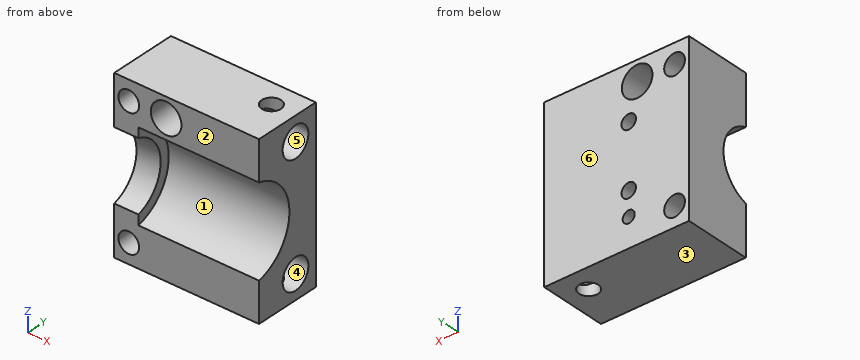
Autodesk Inventor part; units mm, degrees
ref_plane "YZ Plane" through (0, 0, 0) normal (1, 0, 0) x (0, 1, 0)
ref_plane "XZ Plane" through (0, 0, 0) normal (0, 1, 0) x (-1, 0, 0)
ref_plane "XY Plane" through (0, 0, 0) normal (0, 0, 1) x (1, 0, 0)
sketch "Sketch1" plane through (0, 0, 0) normal (0, 0, 1) x (1, 0, 0)
  line L0 (15, -7) -> (-15, -7)
  line L1 (-15, -7) -> (-15, 7)
  line L2 (-15, 7) -> (15, 7)
  line L3 (15, 7) -> (15, -7)
  line L4 (15, -7) -> (-15, 7) construction
  line L5 (-15, -7) -> (15, 7) construction
  point P0 (0, 0)
  dimension "d0" = 30
  dimension "d1" = 14
extrude "Extrusion1" add sketch "Sketch1" along normal blind 35
sketch "Sketch3" plane through (15, -7, 0) normal (1, 0, 0) x (0, 0, -1)
  line L0 (0, 0) -> (-35, 0)
  line L1 (-17.5, 0) -> (-17.5, -2)
  arc A0 (-8.2129, 0) -> (-26.7871, 0) centre (-17.5, -2) ccw
  point P0 (0, 7)
  dimension "d4" = 2
  dimension "d5" = 19
extrude "Extrusion2" cut sketch "Sketch3" against normal blind 25
sketch "Sketch5" plane through (-15, 7, 0) normal (0, 1, 0) x (1, 0, 0)
  line L0 (30, 0) -> (0, 0)
  line L1 (30, -35) -> (0, -35)
  line L2 (0, -35) -> (0, -30.9)
  line L3 (0, 0) -> (0, -35)
  line L4 (0, -30.9) -> (2.75, -30.9)
  circle A0 centre (2.75, -30.9) radius 2
  line L5 (0, 0) -> (0, -4.1)
  line L6 (0, -4.1) -> (2.75, -4.1)
  circle A1 centre (2.75, -4.1) radius 2
  line L7 (2.75, -30.9) -> (10.75, -30.9)
  circle A2 centre (10.75, -30.9) radius 3.175
  point P0 (15, 0)
  dimension "d11" = 4.1
  dimension "d12" = 2.75
  dimension "d13" = 4
  dimension "d14" = 4.1
  dimension "d15" = 2.75
  dimension "d16" = 4
  dimension "d17" = 8
  dimension "d18" = 6.35
extrude "Extrusion3" cut sketch "Sketch5" against normal blind 100 contours A2
sketch "Sketch6" plane through (-15, 7, 0) normal (0, 1, 0) x (1, 0, 0)
  point P0 (15, 0)
sketch "Sketch7" plane through (15, -7, 0) normal (1, 0, 0) x (0, 0, -1)
  line L0 (0, 14) -> (-35, 14)
  line L1 (-35, 14) -> (-30, 14)
  line L2 (-30, 14) -> (-30, 9)
  line L3 (0, 14) -> (0, 0)
  line L4 (0, 14) -> (-5, 14)
  line L5 (-5, 14) -> (-5, 9)
  circle A0 centre (-30, 9) radius 3.175
  circle A1 centre (-5, 9) radius 3.175
  point P0 (0, 7)
  dimension "d21" = 5
  dimension "d22" = 5
  dimension "d23" = 5
  dimension "d24" = 5
  dimension "d25" = 6.35
  dimension "d26" = 6.35
extrude "Extrusion4" cut sketch "Sketch7" against normal blind 15
move or copy body "Move Body1" bodies to move or copy 1 copy no translate (-20, 0, 0)
move or copy body "Move Body2" bodies to move or copy 1 copy no translate (-5, 0, 0)
sketch "Sketch8" plane through (0, 0, 0) normal (1, 0, 0) x (0, 1, 0)
  point P0 (0, 0)
sketch "Sketch9" plane through (-40, 7, 0) normal (0, 1, 0) x (1, 0, 0)
  line L0 (30, -35) -> (0, -35)
  line L1 (0, -35) -> (0, -30.9)
  line L2 (0, 0) -> (0, -35)
  line L3 (0, -30.9) -> (3, -30.9)
  circle A0 centre (3, -30.9) radius 2.15
  line L4 (0, 0) -> (0, -4.1)
  line L5 (0, -4.1) -> (3, -4.1)
  circle A1 centre (3, -4.1) radius 2.15
  point P0 (40, 0)
  dimension "d35" = 4.1
  dimension "d36" = 3
  dimension "d37" = 4.3
  dimension "d38" = 4.1
  dimension "d39" = 4.3
  dimension "d40" = 3
extrude "Extrusion5" cut sketch "Sketch9" against normal blind 14
sketch "Sketch14" plane through (-40, 7, 35) normal (0, 0, 1) x (1, 0, 0)
  line L0 (30, 0) -> (0, 0)
  line L1 (30, 0) -> (25, 0)
  line L2 (25, 0) -> (25, -5)
  circle A0 centre (25, -5) radius 2
  point P0 (40, -7)
  dimension "d47" = 5
  dimension "d48" = 5
  dimension "d49" = 4
extrude "Extrusion6" cut sketch "Sketch14" against normal blind 3
sketch "Sketch15" plane through (-10, 7, 0) normal (0, 0, -1) x (-1, 0, 0)
  line L0 (0, -14) -> (0, 0)
  line L1 (0, 0) -> (5, 0)
  line L2 (0, 0) -> (30, 0)
  line L3 (5, 0) -> (5, -5)
  circle A0 centre (5, -5) radius 2
  point P0 (-10, -7)
  dimension "d52" = 5
  dimension "d53" = 5
  dimension "d54" = 4
extrude "Extrusion7" cut sketch "Sketch15" against normal blind 4
thread "Thread3"
thread "Thread4"
sketch "Sketch16" plane through (-40, -7, 0) normal (-1, 0, 0) x (0, 0, 1)
  line L0 (0, 14) -> (35, 14)
  line L1 (0, 14) -> (17.5, 14)
  line L2 (17.5, 14) -> (17.5, -2)
  circle A0 centre (17.5, -2) radius 7.5
  point P0 (0, 7)
  dimension "d61" = 16
  dimension "d62" = 15
extrude "Extrusion8" cut sketch "Sketch16" against normal blind 15
move or copy body "Move Body3" bodies to move or copy 1 copy no translate (25, 0, 0)
move or copy body "Move Body4" bodies to move or copy 1 copy no translate (10, 0, -15)
move or copy body "Move Body5" bodies to move or copy 1 copy no translate (-10, 0, 0)
sketch "Sketch17" plane through (15, -7, -15) normal (1, 0, 0) x (0, 0, -1)
  point P0 (-15, 7)
sketch "Sketch19" plane through (-15, 7, -15) normal (0, 1, 0) x (1, 0, 0)
  line L0 (30, 0) -> (0, 0)
  line L1 (0, 0) -> (0, -6)
  line L2 (0, 0) -> (6, 0) construction
  line L3 (0, -6) -> (12.5, -6)
  circle A0 centre (12.5, -6) radius 1.25
  line L4 (12.5, -6) -> (12.5, -8.5)
  line L5 (12.5, -6) -> (15, -6) construction
  point P0 (15, -15)
  dimension "d74" = 6
  dimension "d75" = 90
  dimension "d76" = 12.5
  dimension "d77" = 90
  dimension "d78" = 2.5
  dimension "d84" = 2.5
  dimension "d85" = 90
extrude "Extrusion9" cut sketch "Sketch19" against normal blind 12.5
sketch "Sketch20" plane through (-15, 7, -15) normal (0, 1, 0) x (1, 0, 0)
  circle A0 centre (12.5, -6) radius 1.25
  line L0 (12.5, -6) -> (12.5, -11)
  circle A1 centre (12.5, -11) radius 1.5
  line L1 (30, 0) -> (0, 0)
  line L2 (12.5, -11) -> (25.5, -11) construction
  line L3 (0, 0) -> (0, -35)
  line L4 (0, -17.5) -> (30, -17.5)
  line L5 (30, -8.2129) -> (30, -26.7871)
  circle A2 centre (12.5, -24) radius 1.5
  point P0 (15, -15)
  dimension "d86" = 5
  dimension "d87" = 3
extrude "Extrusion10" cut sketch "Sketch20" against normal blind 6 contours A1 | A2
thread "Thread5"
thread "Thread6"
equation "\"d55\" = d54"
properties part number "Rb oven housing top-back" material "Copper"
Verification items for the finished model (mm, model axes). Face numbers are marked on the shaded views. A direction names the side the tool comes from. Coordinates: 2 decimals unless noted, no trailing zeros. Order: outer loops, then holes, each group sorted by start corner. A loop starts at its lowest first (then second) coordinate and runs counter-clockwise, first axis right, second up. Notation, with made-up numbers: M 8.25,77 L 45.25,77 A19 ccw 45.25,93 Z; hole C 16,-30 d1. An arc over 180 degrees is marked long. Write each question's results on one line, items separated by ' | '.
1) Section check C-C on y = -4.75. Record the cut outline in (x, z) (3 decimals), plus the area to 3 significant figures.
Solved:
outline: M -15,-15 L 15,-15 L 15,-5.996 L -10,-5.996 L -10,-3.68 L -15,-3.68 Z; M -15,8.68 L -10,8.68 L -10,10.996 L 15,10.996 L 15,20 L -15,20 Z; hole C -12,-10.9 d4.3; hole C -12,15.9 d4.3; hole C -4.25,15.9 d6.35; hole C -2.5,-9 d2.5 | area: 498 mm²
2) Gauge pin test, flat ends, axial feed: pin 1 Ø4.5 at (x, y) = (10, 2) entering from +Z; pin 2 Ø3.5 at (x, y) = (10, 2) entering from -Z; pin 3 Ø1 at (x, y) = (10, 3) entering from +Z; pin 4 Ø2.5 at (x, z) = (-12, 15.9) entering from -Y. Record the tip position at first contact, or that the pin passes through.
Solved:
pin 1: stops at z = 20 | pin 2: stops at z = -7.35 | pin 3: stops at z = 12.2 | pin 4: passes through
3) Section check A-A on y = 6. Record the cut outline in (x, z) (3 decimals), plus the area to 3 significant figures.
Solved:
outline: M -15,-15 L 15,-15 L 15,20 L -15,20 Z; hole C -12,-10.9 d4.3; hole C -12,15.9 d4.3; hole C -4.25,15.9 d6.35; hole C -2.5,-4 d3; hole C -2.5,9 d3; hole C -2.5,-9 d2.5 | area: 970 mm²
4) Scan lines: line 1 along Z through (x, y) = (-12, 1); line 2 along Z through (x, y) = (5.25, 2) (3 decimals); line 3 along Y through (x, z) = (11, 15) (3 decimals). Record each from-to range of solid material in increasing order. Write a range as [from, to].
Solved:
line 1: z = [-15, -13.05], [-8.75, 13.75], [18.05, 20] | line 2: z = [-15, -13.175], [-6.825, 11.825], [18.175, 20] | line 3: y = [-7, -1.175], [5.175, 7]
5) Section check D-D on x = -2.5. Record the cut outline in (y, z).
Solved:
outline: M -7,-15 L 7,-15 L 7,-10.25 L -5.5,-10.25 L -5.5,-7.75 L 7,-7.75 L 7,-5.5 L 1,-5.5 L 1,-2.5 L 7,-2.5 L 7,7.5 L 1,7.5 L 1,10.5 L 7,10.5 L 7,13.25 L -7,13.25 L -7,11.79 A9.5 cw -7,-6.79 Z; M -7,18.55 L 7,18.55 L 7,20 L -7,20 Z
6) Section check B-B on x = 13. Record the cut outline in (y, z) (3 decimals), plus the area to 3 significant figures.
Solved:
outline: M -7,-15 L 7,-15 L 7,20 L -7,20 L -7,11.787 A9.5 cw -7,-6.787 Z; hole C 2,-10 d6.35; hole C 2,15 d6.35 | area: 323 mm²
7) Access from +Z, -Z, +X, -X, +Y, -Y to the whole of each face (thin tool, end or side, straight path). Record for the marked faces 1 and 2.
Solved:
face 1: +X, -Y | face 2: +Z, -Z, +X, -X, -Y
8) Release check for a two-part mould opening along Y. For the marked faces 3, 4, 5 and 6 record: pulls with the +Y half, pulls with the -Y half, needs draft (parallel to the pull), parting line crosses it, or undercut.
Solved:
face 3: needs draft | face 4: undercut | face 5: undercut | face 6: pulls with the +Y half
